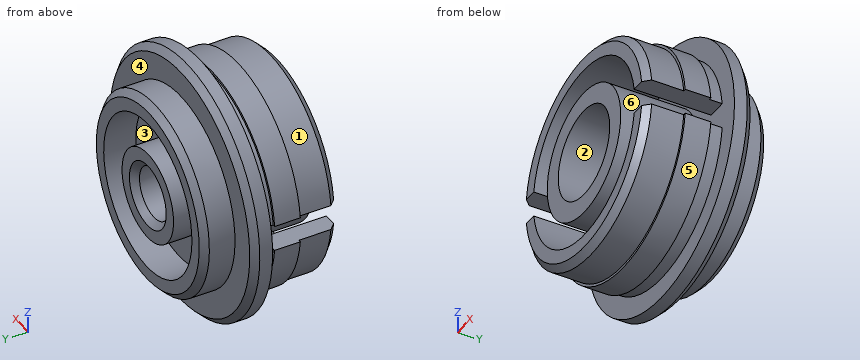
from build123d import *

# Parameters (mm, degrees)
SKETCH_2_R          = 6
SKETCH_2_R_2        = 3.5
CUT_EXTRUDE_1_DEPTH = 2.5
SKETCH_3_R          = 6.9
SKETCH_3_R_2        = 5
CUT_EXTRUDE_2_DEPTH = 6
CUT_EXTRUDE_START   = -6
SKETCH_4_R          = 3.5
CUT_EXTRUDE_3_DEPTH = 6
CUT_EXTRUDE_4_REACH = 19.321
SKETCH_5_R          = 2
CUT_EXTRUDE_5_DEPTH = 6
CHAMFER_1_SIZE      = 0.5


with BuildPart() as part:
    # 草图1 → 旋转1 (revolve)
    with BuildSketch(Plane.XY, mode=Mode.PRIVATE) as revolve_1_sk:
        Polygon((0, 0), (7.5, 0), (7.5, -2.5), (10, -2.5), (10, -4), (8.4, -4), (8.4, -5), (8.6, -5), (8.6, -7), (8.4, -7), (8.4, -10), (0, -10), align=None)
    revolve(revolve_1_sk.sketch.rotate(Axis((0, -10, 0), (0, 1, 0)), 90), axis=Axis((0, -10, 0), (0, 1, 0)))

    # 草图2 → 切除-拉伸1 (cut)
    with BuildSketch(Plane(origin=(0, 0, 0), x_dir=(1, 0, 0), z_dir=(0, 1, 0))):
        with Locations(Location((0, 0, 0), (0, 0, 270))):
            Circle(SKETCH_2_R)
        with Locations(Location((0, 0, 0), (0, 0, 270))):
            Circle(SKETCH_2_R_2, mode=Mode.SUBTRACT)
    extrude(amount=-CUT_EXTRUDE_1_DEPTH, mode=Mode.SUBTRACT)

    # 草图3 → 切除-拉伸2 (cut)
    with BuildSketch(Plane.XZ.offset(10)):
        with Locations(Location((0, 0, 0), (0, 0, 270))):
            Circle(SKETCH_3_R)
        with Locations(Location((0, 0, 0), (0, 0, 270))):
            Circle(SKETCH_3_R_2, mode=Mode.SUBTRACT)
    extrude(amount=-CUT_EXTRUDE_2_DEPTH, mode=Mode.SUBTRACT)

    # 草图4 → 切除-拉伸3 (cut)
    with BuildSketch(Plane.XZ.offset(10).offset(CUT_EXTRUDE_START)):
        with Locations(Location((0, 0, 0), (0, 0, 90))):
            Circle(SKETCH_4_R)
    extrude(amount=CUT_EXTRUDE_3_DEPTH, mode=Mode.SUBTRACT)

    # 草图5 → 切除-拉伸4 (cut, up to next)
    with BuildSketch(Plane(origin=(0, 0, 0), x_dir=(1, 0, 0), z_dir=(0, 1, 0)), mode=Mode.PRIVATE) as cut_extrude_4_sk1:
        with Locations(Location((0, 0, 0), (0, 0, 270))):
            Circle(SKETCH_5_R)
    cut_extrude_4_tool1 = extrude(cut_extrude_4_sk1.sketch, amount=-CUT_EXTRUDE_4_REACH, mode=Mode.PRIVATE) & part.part
    add(cut_extrude_4_tool1.solids().sort_by_distance((0, 0, 0))[0], mode=Mode.SUBTRACT)

    # 草图6 → 切除-拉伸5 (cut)
    with BuildSketch(Plane.XZ.offset(10).offset(CUT_EXTRUDE_START)):
        with BuildLine():
            Line((-8.94427191, -1), (-5.916079783, -1))
            ThreePointArc((-5.916079783, -1), (-6, 0), (-5.916079783, 1))
            Line((-5.916079783, 1), (-8.94427191, 1))
            ThreePointArc((-8.94427191, 1), (-9, 0), (-8.94427191, -1))
        make_face()
        with BuildLine():
            Line((5.916079783, 1), (8.94427191, 1))
            ThreePointArc((8.94427191, 1), (9, 0), (8.94427191, -1))
            Line((8.94427191, -1), (5.916079783, -1))
            ThreePointArc((5.916079783, -1), (6, 0), (5.916079783, 1))
        make_face()
    extrude(amount=CUT_EXTRUDE_5_DEPTH, mode=Mode.SUBTRACT)

    # 倒角1
    chamfer_1_edges = [part.edges().sort_by_distance(p)[0] for p in [
        (0, -2.5, 10),
        (0, 0, 7.5),
        (0, 0, -2),
        (0, -10, -8.4),
        (0, -10, 8.4),
    ]]
    chamfer(chamfer_1_edges, length=CHAMFER_1_SIZE)


solid = part.part
Here's how the part is built. I have some questions about the finished solid (model axes, mm). Face numbers are marked on the shaded views. A direction names the side the tool comes from. Round coordinates to 2 decimals unless told otherwise and drop trailing zeros. Loops run counter-clockwise (first coordinate to the right, second up) from the corner with the lowest first, then second, coordinate; pieces in that order, holes last. Notation, with made-up numbers: (66.25, -24) - (118.25, -24) arc R19 ccw to (118.25, 7) - close; hole circle Ø7 at (89, 52.5). An arc over 180 degrees is marked (long way). One line per question, with ' | ' between items. Start each with the question number.
Q1. I want a section at A-A (y = -7.75). Write out the boundary of the cut face in (x, z).
Q2. For the marked faces 1, 2 and 3, which set-ups out of +Z, -Z, +X, -X, +Y, -Y let a thin tool reach every point of the face, with its end or its side?
Q3. We'd pull the mould along X, two halves only. Please class the marked faces 4, 5 and 6: +X half, -X half, draft (parallel to the pull), parting line (faces both ways), or undercut.
Q4. Will these pins go through, and if not, where does the flat tip stop? pin 1 (4 mm diameter, centred on x = -3.5, y = -5, fed in from +Z); pin 2 (1.9 mm diameter, centred on x = -7.5, y = -6, fed in from -Z); pin 3 (0.9 mm diameter, centred on x = 7.5, y = -7.5, fed in from +Z).
Q5. Please list where these lines run through material, in increasing order: line 1 (X direction, y = -1.4, z = 0); line 2 (Y direction, x = -6.75, z = 5.25); line 3 (Z direction, x = 1, y = -7.25). Write a range as [from, to].
Q6. I want a section at C-C (y = -2). Write out the boundary of the cut face in (x, z).
Response values:
1) outline: (-8.34, -1) arc R8.4 ccw to (8.34, -1) - (6.83, -1) arc R6.9 cw to (-6.83, -1) - close; (-8.34, 1) - (-6.83, 1) arc R6.9 cw to (6.83, 1) - (8.34, 1) arc R8.4 ccw to start; circle Ø10 at (0, 0); hole circle Ø7 at (0, 0)
2) face 1: +Z, -Y | face 2: -Y | face 3: +Y
3) face 4: draft | face 5: parting line | face 6: undercut
4) pin 1: stops at z = 9.84 | pin 2: stops at z = -5.57 | pin 3: stops at z = 4.57
5) line 1: x = [-7.5, -6], [-3.5, -2], [2, 3.5], [6, 7.5] | line 2: y = [-7, -5], [-4, -2.5] | line 3: z = [-8.34, -6.83], [-4.9, -3.35], [3.35, 4.9], [6.83, 8.34]
6) outline: circle Ø15 at (0, 0); circle Ø7 at (0, 0); hole circle Ø12 at (0, 0); hole circle Ø4 at (0, 0)
